Can you work these out from the model? Positions are in its coordinate system, mm. Give positions to 0.01 mm unless a question says otherwise; leave off trailing zeros. Order: outer loops, then holes, each group sorted by start corner. A loop starts at its lowest first (then second) coordinate and runs counter-clockwise, first axis right, second up. Notation, with made-up numbers: (58.5, -0.5) - (79.5, -0.5) arc R15 cw to (79.5, 22.5) - close; hole circle Ø11 at (-3, 80). An arc over 180 degrees is marked (long way). Answer as a JSON object with one key per item and string values.
Autodesk Inventor part; units mm, degrees
ref_plane "Arbeitsebene2" through (-21.5666, -16.2656, 21.7) normal (0, 0, 1) x (0.7071, -0.7071, 0)
ref_plane "YZ Plane" through (0, 0, 0) normal (1, 0, 0) x (0, 1, 0)
ref_plane "XZ Plane" through (0, 0, 0) normal (0, 1, 0) x (-1, 0, 0)
ref_plane "Arbeitsebene1" through (0, 0, 0) normal (0, 0, 1) x (1, 0, 0)
sketch "Skizze1" plane through (0, 0, 0) normal (0, 0, 1) x (1, 0, 0)
  circle A0 centre (-9.9998, 17.4978) radius 1.3999
  circle A1 centre (10.0001, 17.4979) radius 1.4
  circle A2 centre (10.0001, -17.5021) radius 1.4
  circle A3 centre (-9.9999, -17.5021) radius 1.4001
  circle A4 centre (4.4725, 20.2023) radius 1.4
  circle A5 centre (19.4212, 5.2535) radius 1.4
  circle A6 centre (0.0001, -0.0022) radius 6.7754
  arc A7 (-25.1198, 6.6998) -> (-24.1417, 5.4917) centre (-24.1417, 6.4917) ccw
  line L0 (-24.1417, 5.4917) -> (-17.7002, 5.4917)
  arc A8 (-15.7002, 3.4917) -> (-17.7002, 5.4917) centre (-17.7002, 3.4917) ccw
  line L1 (-15.7002, 3.4917) -> (-15.7002, -4.496)
  arc A9 (-17.7002, -6.496) -> (-15.7002, -4.496) centre (-17.7002, -4.496) ccw
  line L2 (-17.7002, -6.496) -> (-23.8502, -6.496)
  arc A10 (-23.8502, -6.496) -> (-24.8235, -7.7254) centre (-23.8502, -7.496) ccw
  arc A11 (-24.8235, -7.7254) -> (-25.1198, 6.6998) centre (0, 0) ccw
  circle A12 centre (-9.4998, -11.0022) radius 2.6601
  circle A13 centre (-16.8291, -16.0481) radius 1.4
  circle A14 centre (6.1284, 23.0202) radius 1.4
  circle A15 centre (22.7119, 7.1872) radius 1.4
  arc A16 (-25.1198, 6.6998) -> (-24.6232, -8.3421) centre (0, 0) ccw
  circle A17 centre (-9.4998, -11.0022) radius 4.196
  point P0 (0, 0)
ref_plane "Arbeitsebene2" through (-21.5666, -16.2656, 21.7) normal (0, 0, 1) x (0.7071, -0.7071, 0)
extrude "Extrusion1" add sketch "Skizze1" along normal up to surface (21.7 mm away) contours A11 A10 L2 A9 L1 A8 L0 A7 | A7 L0 A8 L1 A9 L2 A10 A16
sketch "Skizze2" plane through (-24.1417, 5.4917, 21.7) normal (0, 0, 1) x (1, 0, 0)
  arc A0 (30.5656, -11.7979) -> (31.153, -11.2105) centre (30.5058, -11.1507) ccw
  line L0 (30.5656, -11.7979) -> (24.8489, -17.5146)
  line L1 (24.8489, -17.5146) -> (19.6708, -12.3365)
  arc A1 (17.2991, -9.9648) -> (19.6708, -12.3365) centre (18.1314, -11.5042) ccw
  line L2 (17.2991, -9.9648) -> (12.8281, -5.4938)
  line L3 (12.8281, -5.4938) -> (15.7017, -2.6202)
  arc A2 (17.7327, -0.5892) -> (15.7017, -2.6202) centre (16.0101, -0.8976) ccw
  line L4 (17.7327, -0.5892) -> (24.1418, 5.8199)
  line L5 (24.1418, 5.8199) -> (28.7374, 1.2243)
  arc A3 (30.8599, -0.8982) -> (28.7374, 1.2243) centre (30.435, 0.7994) ccw
  line L6 (30.8599, -0.8982) -> (36.1626, -6.2009)
  line L7 (36.1626, -6.2009) -> (34.5533, -7.8102)
  arc A4 (32.1151, -10.2485) -> (34.5533, -7.8102) centre (33.5463, -9.2415) ccw
  line L8 (32.1151, -10.2485) -> (31.153, -11.2105)
  circle A5 centre (12.8281, -4.0796) radius 0.65
  line L9 (21.2427, 4.9006) -> (17.8485, 8.2948)
  line L10 (17.8485, 8.2948) -> (14.4544, 11.6889)
  line L11 (14.4544, 11.6889) -> (2.575, -0.1905)
  line L12 (2.575, -0.1905) -> (24.1418, -21.7573)
  line L13 (24.1418, -21.7573) -> (42.8094, -3.0897)
  line L14 (42.8094, -3.0897) -> (28.0309, 11.6889)
  line L15 (28.0309, 11.6889) -> (24.6368, 8.2948)
  line L16 (24.6368, 8.2948) -> (21.2427, 4.9006)
  circle A6 centre (21.2427, 11.6889) radius 4.8
  line L17 (42.8094, -3.0897) -> (24.1418, -21.7573)
  line L18 (24.1418, -21.7573) -> (2.575, -0.1905)
  line L19 (2.575, -0.1905) -> (21.2427, 18.4771)
  line L20 (21.2427, 18.4771) -> (42.8094, -3.0897)
  line L21 (21.2427, 19.1842) -> (1.8679, -0.1905)
  line L22 (1.8679, -0.1905) -> (24.1418, -22.4644)
  line L23 (24.1418, -22.4644) -> (43.5165, -3.0897)
  line L24 (43.5165, -3.0897) -> (21.2427, 19.1842)
  point P0 (24.1417, -5.4917)
  dimension "d2" = 0.5
extrude "Extrusion2" cut sketch "Skizze2" against normal through all contours L0 L1 A1 L2 L3 A2 L4 L5 A3 L6 L7 A4 L8 A0 | A5 | L16 L15 L14 L13 L12 L11 L10 L9 | L9 A6 L16 | A6 | L10 L19 A6 | A6 L20 L15 | L19 L20 A6 | L24 L23 L22 L21
fillet "Rundung1" radius 1 8 edges at (-2.899, 24.6759, 10.85) (19.3748, 2.402, 10.85) (0.0001, -16.9727, 10.85) (-22.2737, 5.3011, 10.85) (-10.1203, -6.8523, 10.85) (-5.3499, -11.6226, 10.85) (-11.0276, 16.5473, 10.85) (-9.0493, 18.5256, 10.85)
properties part number "Matchboxscope_focusingblock_v0"
Q1. If we section it at B-B, the plane z = 6.5: Count the separate pieces of the cut face and the enclosed holes in it, then the cut area to 3 significant figures.
Recorded:
{"separate pieces": "1", "enclosed holes": "9", "area": "1,160 mm^2"}
Q2. We'd pull the mould along X, two halves only. Please class faces 1 (the face through (-21.86, 5.29, 10.7)), 2 (the face through (25.95, 1.57, 10.7)), 3 (the face through (-25.99, -0.64, 10.7)): released by +X, released by -X, zero draft, split by the parting line, or undercut.
Recorded:
{"face 1": "undercut", "face 2": "split by the parting line", "face 3": "released by -X"}
Q3. If we section it at A-A, the plane x = 22: Please give me the cut outline in (y, z).
Recorded:
{"outline": "(-13.85, 0) - (5.98, 0) - (5.98, 21.7) - (-13.85, 21.7) - close; (8.39, 0) - (13.85, 0) - (13.85, 21.7) - (8.39, 21.7) - close"}
Q4. If we section it at C-C, the plane y = -8.5: Please give me the cut outline in (x, z), then the cut area to 3 significant figures.
Recorded:
{"outline": "(-24.57, 0) - (-12.87, 0) - (-12.87, 21.7) - (-24.57, 21.7) - close; (8.47, 0) - (24.57, 0) - (24.57, 21.7) - (8.47, 21.7) - close", "area": "603 mm^2"}
Q5. I need wall thicknesses on L1, parallel to X at y = 6, z = 18.75; L2, parallel to X at y = -16, z = 9.5; L3, parallel to Y at x = -17.5, z = 18.5. Which ranges of each line are inside material? Lowest first, please.
Recorded:
{"L1": "x = -25.3 to -21.57, 15.78 to 18.24, 20.61 to 21.97, 23.45 to 25.3", "L2": "x = -20.49 to -18.23, -15.43 to -0.97, 0.97 to 20.49", "L3": "y = -19.23 to -17.28, -14.82 to 0.53, 10.07 to 19.23"}
Q6. I'm going to push flat-ended pins straight in: pin 1 Ø3 at (x, z) = (-18, 19.5) entering from -Y; pin 2 Ø2 at (x, y) = (4.47, 20.2) entering from -Z; pin 3 Ø1 at (x, z) = (12, 10.5) entering from -Y; pin 4 Ø1 at (y, z) = (13, 7) entering from -X. Where does each tip first touch, or does it pass through?
Recorded:
{"pin 1": "stops at y = -20.09", "pin 2": "passes through", "pin 3": "stops at y = -23.32", "pin 4": "stops at x = -22.8"}
